Check sheet for the modelled part. Datum: model origin and axes. Units: mm. Face numbers are marked on the shaded views. A direction names the side the tool comes from. Round coordinates to 2 decimals unless told otherwise and drop trailing zeros. Write each loop counter-clockwise with the first axis right and the second up, starting at its lowest first coordinate (ties: lowest second). Pieces come first, ordered by that corner, then holes.
Item 1: Section check A-A, the plane x = 0. Record the cut outline in (y, z), plus the area to 3 significant figures.
Item 2: Section check B-B, the plane z = 2.5. Record the cut outline in (x, y).
Item 3: Set-up check for the marked faces 1 and 2: record each of +Z, -Z, +X, -X, +Y, -Y from which the full face is reachable in a straight line by a thin tool's end or side.
Item 4: Section check D-D, the plane z = -36. Record the cut outline in (x, y), plus the area to 3 significant figures.
Item 5: Depth check by flat-ended pin: pin 1 (4 mm diameter, centred on x = -27, y = 18.5, fed in from +Z); pin 2 (8 mm diameter, centred on x = -57, y = 14, fed in from +Z); pin 3 (4 mm diameter, centred on x = -26, y = 21.5, fed in from -Z); pin 4 (13 mm diameter, centred on x = 0, z = -40, fed in from -Y). Enter the tip coordinate at first touch or a pass-through.
Item 6: Material ranges on line 1 along X through (y, z) = (5.25, 0); line 2 along Z through (x, y) = (-0.5, 15.75) (3 decimals); line 3 along Z through (x, y) = (-7.5, 19), recorded low to high.
Item 7: Release check for a two-part mould opening along Z. For the marked faces 3, 4 and 5 record: pulls with the +Z half, pulls with the -Z half, needs draft (parallel to the pull), parting line crosses it, or undercut.
Item 8: Section check C-C, the plane y = 14.75. Record the cut outline in (x, z).
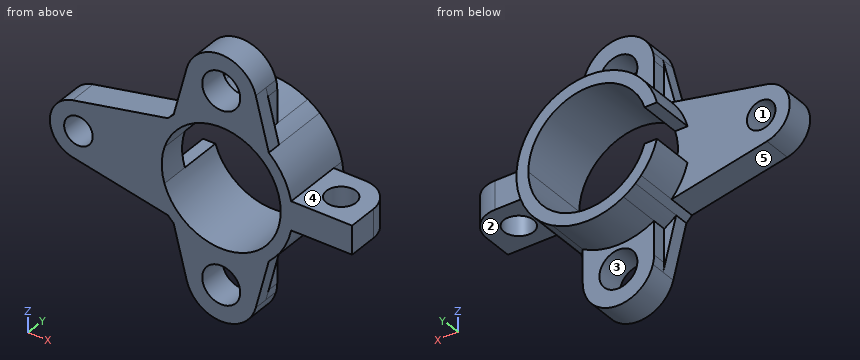
from build123d import *

# Parameters (mm, degrees)
Y_KSEKLIK_EKSTR_ZYON2_DEPTH = 30
IZIM1_7_R                   = 6
IZIM1_7_R_2                 = 7.987749768
Y_KSEKLIK_EKSTR_ZYON3_DEPTH = 12
Y_KSEKLIK_EKSTR_ZYON6_DEPTH = 6
Y_KSEKLIK_EKSTR_ZYON7_DEPTH = 25
RADYUS1_R                   = 12.5
IZIM2_R                     = 6.25
KES_EKSTR_ZYON1_DEPTH       = 61.978720201


with BuildPart() as part:
    # izim1 → Y_kseklik-Ekstr_zyon2 (new body)
    with BuildSketch(Plane(origin=(0, 0, 0), x_dir=(1, 0, 0), z_dir=(0, 1, 0))):
        with BuildLine():
            ThreePointArc((-20, 22.360679775), (-21.213203436, 21.213203436), (-22.360679775, 20))
            ThreePointArc((-22.360679775, 20), (-26.452968197, 14.150635095), (-29.047375097, 7.5))
            Line((-29.047375097, 7.5), (-23.848480035, 7.5))
            ThreePointArc((-23.848480035, 7.5), (3.793942482, 24.710443145), (25, 0))
            ThreePointArc((25, 0), (3.793942482, -24.710443145), (-23.848480035, -7.5))
            Line((-23.848480035, -7.5), (-29.047375097, -7.5))
            ThreePointArc((-29.047375097, -7.5), (-26.452968197, -14.150635095), (-22.360679775, -20))
            ThreePointArc((-22.360679775, -20), (-21.213203436, -21.213203436), (-20, -22.360679775))
            ThreePointArc((-20, -22.360679775), (-17.58340753, -24.306866923), (-14.978720201, -25.993036397))
            ThreePointArc((-14.978720201, -25.993036397), (0, -30), (14.978720201, -25.993036397))
            ThreePointArc((14.978720201, -25.993036397), (17.58340753, -24.306866923), (20, -22.360679775))
            ThreePointArc((20, -22.360679775), (26.016470356, -14.937980794), (29.393876913, -6))
            ThreePointArc((29.393876913, -6), (30, 0), (29.393876913, 6))
            ThreePointArc((29.393876913, 6), (26.016470356, 14.937980794), (20, 22.360679775))
            ThreePointArc((20, 22.360679775), (17.58340753, 24.306866923), (14.978720201, 25.993036397))
            ThreePointArc((14.978720201, 25.993036397), (0, 30), (-14.978720201, 25.993036397))
            ThreePointArc((-14.978720201, 25.993036397), (-17.58340753, 24.306866923), (-20, 22.360679775))
        make_face()
    extrude(amount=Y_KSEKLIK_EKSTR_ZYON2_DEPTH)

    # izim1_7 → Y_kseklik-Ekstr_zyon3 (add)
    with BuildSketch(Plane(origin=(0, 0, 0), x_dir=(1, 0, 0), z_dir=(0, 1, 0))):
        with BuildLine():
            Line((-22.360679775, 20), (-62.419565489, 11.753540013))
            ThreePointArc((-62.419565489, 11.753540013), (-72, 0), (-62.419565489, -11.753540013))
            Line((-62.419565489, -11.753540013), (-22.360679775, -20))
            ThreePointArc((-22.360679775, -20), (-26.452968197, -14.150635095), (-29.047375097, -7.5))
            Line((-29.047375097, -7.5), (-23.848480035, -7.5))
            ThreePointArc((-23.848480035, -7.5), (-25, 0), (-23.848480035, 7.5))
            Line((-23.848480035, 7.5), (-29.047375097, 7.5))
            ThreePointArc((-29.047375097, 7.5), (-26.452968197, 14.150635095), (-22.360679775, 20))
        make_face()
        with Locations((-60, 0)):
            Circle(IZIM1_7_R, mode=Mode.SUBTRACT)
        with BuildLine():
            ThreePointArc((-14.978720201, -40), (-14.860343614, -41.879427184), (-14.507084908, -43.729148203))
            ThreePointArc((-14.507084908, -43.729148203), (0, -54.978720201), (14.507084908, -43.729148203))
            ThreePointArc((14.507084908, -43.729148203), (14.860343614, -41.879427184), (14.978720201, -40))
            Line((14.978720201, -40), (14.978720201, -25.993036397))
            ThreePointArc((14.978720201, -25.993036397), (0, -30), (-14.978720201, -25.993036397))
            Line((-14.978720201, -25.993036397), (-14.978720201, -40))
        make_face()
        with Locations((0, -40)):
            Circle(IZIM1_7_R_2, mode=Mode.SUBTRACT)
        with BuildLine():
            ThreePointArc((14.507084908, 43.729148203), (0, 54.978720201), (-14.507084908, 43.729148203))
            ThreePointArc((-14.507084908, 43.729148203), (-14.860343614, 41.879427184), (-14.978720201, 40))
            Line((-14.978720201, 40), (-14.978720201, 25.993036397))
            ThreePointArc((-14.978720201, 25.993036397), (0, 30), (14.978720201, 25.993036397))
            Line((14.978720201, 25.993036397), (14.978720201, 40))
            ThreePointArc((14.978720201, 40), (14.860343614, 41.879427184), (14.507084908, 43.729148203))
        make_face()
        with Locations((0, 40)):
            Circle(IZIM1_7_R_2, mode=Mode.SUBTRACT)
    extrude(amount=Y_KSEKLIK_EKSTR_ZYON3_DEPTH)

    # izim1_12 → Y_kseklik-Ekstr_zyon6 (add)
    with BuildSketch(Plane(origin=(0, 0, 0), x_dir=(1, 0, 0), z_dir=(0, 1, 0))):
        with BuildLine():
            Line((-14.507084908, 43.729148203), (-20, 22.360679775))
            ThreePointArc((-20, 22.360679775), (-17.58340753, 24.306866923), (-14.978720201, 25.993036397))
            Line((-14.978720201, 25.993036397), (-14.978720201, 40))
            ThreePointArc((-14.978720201, 40), (-14.860343614, 41.879427184), (-14.507084908, 43.729148203))
        make_face()
        with BuildLine():
            ThreePointArc((-14.978720201, -25.993036397), (-17.58340753, -24.306866923), (-20, -22.360679775))
            Line((-20, -22.360679775), (-14.507084908, -43.729148203))
            ThreePointArc((-14.507084908, -43.729148203), (-14.860343614, -41.879427184), (-14.978720201, -40))
            Line((-14.978720201, -40), (-14.978720201, -25.993036397))
        make_face()
        with BuildLine():
            ThreePointArc((14.978720201, -40), (14.860343614, -41.879427184), (14.507084908, -43.729148203))
            Line((14.507084908, -43.729148203), (20, -22.360679775))
            ThreePointArc((20, -22.360679775), (17.58340753, -24.306866923), (14.978720201, -25.993036397))
            Line((14.978720201, -25.993036397), (14.978720201, -40))
        make_face()
        with BuildLine():
            Line((20, 22.360679775), (14.507084908, 43.729148203))
            ThreePointArc((14.507084908, 43.729148203), (14.860343614, 41.879427184), (14.978720201, 40))
            Line((14.978720201, 40), (14.978720201, 25.993036397))
            ThreePointArc((14.978720201, 25.993036397), (17.58340753, 24.306866923), (20, 22.360679775))
        make_face()
    extrude(amount=Y_KSEKLIK_EKSTR_ZYON6_DEPTH)

    # izim1_13 → Y_kseklik-Ekstr_zyon7 (add)
    with BuildSketch(Plane(origin=(0, 0, 0), x_dir=(1, 0, 0), z_dir=(0, 1, 0))):
        with BuildLine():
            Line((55, 6), (29.393876913, 6))
            ThreePointArc((29.393876913, 6), (30, 0), (29.393876913, -6))
            Line((29.393876913, -6), (55, -6))
            Line((55, -6), (55, 6))
        make_face()
    extrude(amount=Y_KSEKLIK_EKSTR_ZYON7_DEPTH)

    # Radyus1
    radyus1_edges = [part.edges().sort_by_distance(p)[0] for p in [
        (55, 25, 0),
    ]]
    fillet(radyus1_edges, radius=RADYUS1_R)

    # izim2 → Kes-Ekstr_zyon1 (cut, through all)
    with BuildSketch(Plane.XY.offset(6)):
        with Locations((41.698353051, 12.200101709)):
            Circle(IZIM2_R)
    extrude(amount=-KES_EKSTR_ZYON1_DEPTH, mode=Mode.SUBTRACT)


solid = part.part
Values found:
1. outline: (0, -54.98) - (12, -54.98) - (12, -47.99) - (0, -47.99) - close; (0, -32.01) - (12, -32.01) - (12, -30) - (30, -30) - (30, -25) - (0, -25) - close; (0, 25) - (30, 25) - (30, 30) - (12, 30) - (12, 32.01) - (0, 32.01) - close; (0, 47.99) - (12, 47.99) - (12, 54.98) - (0, 54.98) - close
1. area: 516 mm2
2. outline: (-71.74, 0) - (-65.45, 0) - (-65.45, 12) - (-71.74, 12) - close; (-54.55, 0) - (-24.87, 0) - (-24.87, 12) - (-54.55, 12) - close; (24.87, 0) - (55, 0) - (55, 12.5) arc R12.5 ccw to (42.5, 25) - (29.9, 25) - (29.9, 30) - (24.87, 30) - close; hole circle Ø12.5 at (41.7, 12.2)
3. face 1: +Y, -Y
3. face 2: -Z, +X, +Y, -Y
4. outline: (-16.49, 0) - (-6.91, 0) - (-6.91, 12) - (-14.98, 12) - (-14.98, 6) - (-16.49, 6) - close; (6.91, 0) - (16.49, 0) - (16.49, 6) - (14.98, 6) - (14.98, 12) - (6.91, 12) - close
4. area: 212 mm2
5. pin 1: stops at z = 16.58
5. pin 2: stops at z = 13.58
5. pin 3: stops at z = -18
5. pin 4: passes through
6. line 1: x = -72 to -66, -54 to -25, 25 to 55
6. line 2: z = -29.996 to -24.995, 24.995 to 29.996
6. line 3: z = -29.05 to -23.85, 23.85 to 29.05
7. face 3: undercut
7. face 4: pulls with the +Z half
7. face 5: pulls with the -Z half
8. outline: (-29.05, -7.5) arc R30 ccw to (29.39, -6) - (35.99, -6) - (35.99, 6) - (29.39, 6) arc R30 ccw to (-29.05, 7.5) - (-23.85, 7.5) arc R25 cw (long way) to (-23.85, -7.5) - close; (47.4, -6) - (54.8, -6) - (54.8, 6) - (47.4, 6) - close
